```python
from build123d import *

# Parameters (mm, degrees)
F0_W     = 101.6
F0_H     = 63.5
F1_DEPTH = 76.2
F2_R     = 32.797713
F3_DEPTH = 127
F4_DEPTH = 127


with BuildPart() as f1:
    # F0 (on Front) → F1 (new body)
    with BuildSketch(Plane.XZ):
        with Locations((7.209563, 1.568823)):
            Rectangle(F0_W, F0_H)
    extrude(amount=F1_DEPTH)

    # F2 (on Top) → F3 (cut)
    with BuildSketch(Plane.XY):
        with Locations((37.366524, -38.079627)):
            Circle(F2_R)
    extrude(amount=F3_DEPTH, mode=Mode.SUBTRACT)

    # F3_face (on face) → F4 (cut)
    with BuildSketch(Plane(origin=(33.622944, -38.079627, 0), x_dir=(1, 0, 0), z_dir=(0, 0, 1))):
        with BuildLine():
            Line((24.386619, -25.486367), (24.386619, 25.486367))
            ThreePointArc((24.386619, 25.486367), (-29.054133, 0), (24.386619, -25.486367))
        make_face()
    extrude(amount=-F4_DEPTH, mode=Mode.SUBTRACT)


solid = f1.part
```
Can you work these out from the model? Positions are in its coordinate system, mm. Round coordinates to 2 decimals unless told otherwise and drop trailing zeros. Order: outer loops, then holes, each group sorted by start corner. A loop starts at its lowest first (then second) coordinate and runs counter-clockwise, first axis right, second up. Notation, with made-up numbers: (72.5, -10.5) -> (106.5, -10.5) arc R27 cw to (106.5, 25.5) -> close; hole circle Ø1 at (16.5, 45.5). An arc over 180 degrees is marked (long way). Return JSON: item names as keys, results as strings. Group by question number.
1. I need wall thicknesses on line 1 (Y direction, x = 38, z = 13.5); line 2 (Y direction, x = 25, z = 13); line 3 (X direction, y = -9.5, z = -10.5). Which ranges of each line are inside material? Lowest first, please. Write a range as [from, to].
2. If we section it at B-B, the plane y = -10.5: Write out the boundary of the cut face in (x, z).
3. We'd pull the mould along Y, two halves only. Please class faces 1 (the face through (6, -76.2, 2)), 2 (the face through (-43.59, -38, 1)), 3 (the face through (6, 0, 2)): released by +Y, released by -Y, zero draft, split by the parting line, or undercut.
4. If we section it at A-A, the plane x = 32.5: Write out the boundary of the cut face in (y, z), then the cut area to 4 significant figures.
5. If we section it at C-C, the plane z = 17.5: Write out the boundary of the cut face in (x, y).
6. Will this pin go through, and if not, where does the flat tip stop? pin 1 (1 mm diameter, centred on y = -41.5, z = -11.5, fed in from +X).
7. If we section it at D-D, the plane y = -33: Write out the boundary of the cut face in (x, z).
Output values:
{
 "1": {"line 1": "[-76.2, -70.87], [-5.29, 0]", "line 2": "[-76.2, -68.46], [-7.7, 0]", "line 3": "[-43.59, 21.28], [53.46, 58.01]"},
 "2": {"outline": "(-43.59, -30.18) -> (19.62, -30.18) -> (19.62, 33.32) -> (-43.59, 33.32) -> close; (55.12, -30.18) -> (58.01, -30.18) -> (58.01, 33.32) -> (55.12, 33.32) -> close"},
 "3": {"face 1": "released by -Y", "face 2": "zero draft", "face 3": "released by +Y"},
 "4": {"outline": "(-76.2, -30.18) -> (-70.51, -30.18) -> (-70.51, 33.32) -> (-76.2, 33.32) -> close; (-5.64, -30.18) -> (0, -30.18) -> (0, 33.32) -> (-5.64, 33.32) -> close", "area": "719.5 mm²"},
 "5": {"outline": "(-43.59, -76.2) -> (58.01, -76.2) -> (58.01, -63.57) arc R32.8 cw (long way) to (58.01, -12.59) -> (58.01, 0) -> (-43.59, 0) -> close"},
 "6": {"pin 1": "x = 4.8"},
 "7": {"outline": "(-43.59, -30.18) -> (4.96, -30.18) -> (4.96, 33.32) -> (-43.59, 33.32) -> close"}
}
